CAD build for the part. Positions are in the model's coordinates, mm. A direction names the side the tool comes from. Give positions to 0.01 mm unless a question says otherwise; leave off trailing zeros. Write each loop counter-clockwise with the first axis right and the second up, starting at its lowest first coordinate (ties: lowest second). Pieces come first, ordered by that corner, then holes. Notation, with made-up numbers: (-31.75, -9.5) - (6.25, -9.5) arc R16 ccw to (6.25, 21.5) - close; hole circle Ø6 at (2, 50.5). An arc over 180 degrees is marked (long way). Put each result on its own line as item: value. Start each with the question number.
1. Drop flat-ended pins along their axis: pin 1 (7.5 mm diameter, centred on x = 28.5, z = 5.5, fed in from +Y); pin 2 (7.5 mm diameter, centred on y = 18, z = -2, fed in from +X); pin 3 (6 mm diameter, centred on x = 11, z = 9, fed in from +Y). Give the stop position or say it passes through.
2. Mould opens along Y. For faces 1 (the flat face through (18, 0, 0)), 2 (the cylindrical face through (2.948, 21.418, -0.526)), 3 (the flat face through (6, 9, -19.05)), 4 (the cylindrical face through (7.405, 7.331, 0.267)) say: +Y half, -Y half, draft (parallel to the pull), parting line (faces both ways), or undercut.
3. Cut at C-C on z = -8. List the corners of the cut face in (x, y), and give its area (3 significant figures).
4. Tool access for faces 5 (the flat face through (0, 23, 0)), 6 (the flat face through (5.969, 23, 0)): list every direction of +Z, -Z, +X, -X, +Y, -Y with a clear straight run to the whole face (end or side of a thin tool).
5. Wall check: line 1 (Z direction, x = 3.35, y = 19.05); line 2 (Y direction, x = 4.3, z = 0); line 3 (X direction, y = 10.5, z = 13). Give the ranges that are in metal, low to high.
6. Cut at D-D on y = 14. List the corners of the cut face in (x, z), and give its area (3 significant figures).
7. Cut at B-B on y = 19.05. List the corners of the cut face in (x, z).
8. Cut at A-A on z = 0. List the corners of the cut face in (x, y).
from build123d import *

# Parameters (mm, degrees)
BOSS_EXTRUDE1_DEPTH = 19.05


with BuildPart() as part:
    # Sketch1 → Boss-Extrude1 (new, symmetric)
    with BuildSketch(Plane.XY):
        with BuildLine():
            Line((0, 36.5252), (0, 0))
            Line((0, 0), (36.5252, 0))
            Line((36.5252, 0), (36.5252, 5.969))
            Line((36.5252, 5.969), (10.7442, 5.969))
            ThreePointArc((10.7442, 5.969), (7.367623698, 7.367623698), (5.969, 10.7442))
            Line((5.969, 10.7442), (5.969, 36.5252))
            Line((5.969, 36.5252), (0, 36.5252))
        make_face()
    extrude(amount=BOSS_EXTRUDE1_DEPTH, both=True)

    # Sketch9 → #11 (0.191) Diameter Hole1 (revolve, cut)
    with BuildSketch(Plane.ZX.offset(19.05)):
        Polygon((0, 0), (0, 5.969), (2.794, 5.969), (2.4257, 5.6007), (2.4257, 0.3683), (2.794, 0), align=None)
    revolve(axis=Axis((-6.35, 19.05, 0), (1, 0, 0)), mode=Mode.SUBTRACT)


solid = part.part
Report:
1. pin 1: stops at y = 5.97
1. pin 2: stops at x = 5.97
1. pin 3: stops at y = 6.84
2. face 1: -Y half
2. face 2: undercut
2. face 3: draft
2. face 4: +Y half
3. outline: (0, 0) - (36.53, 0) - (36.53, 5.97) - (10.74, 5.97) arc R4.78 cw to (5.97, 10.74) - (5.97, 36.53) - (0, 36.53) - close
3. area: 405 mm²
4. face 5: +Z, -Z, -X, +Y, -Y
4. face 6: +Z, -Z, +X, +Y
5. line 1: z = -19.05 to -2.43, 2.43 to 19.05
5. line 2: y = 0 to 16.62, 21.48 to 36.53
5. line 3: x = 0 to 5.98
6. outline: (0, -19.05) - (5.97, -19.05) - (5.97, 19.05) - (0, 19.05) - close
6. area: 227 mm²
7. outline: (0, -19.05) - (5.97, -19.05) - (5.97, -2.79) - (5.6, -2.43) - (0.37, -2.43) - (0, -2.79) - close; (0, 2.79) - (0.37, 2.43) - (5.6, 2.43) - (5.97, 2.79) - (5.97, 19.05) - (0, 19.05) - close
8. outline: (0, 0) - (36.53, 0) - (36.53, 5.97) - (10.74, 5.97) arc R4.78 cw to (5.97, 10.74) - (5.97, 16.26) - (5.6, 16.62) - (0.37, 16.62) - (0, 16.26) - close; (0, 21.84) - (0.37, 21.48) - (5.6, 21.48) - (5.97, 21.84) - (5.97, 36.53) - (0, 36.53) - close
